Can you work these out from the model? Positions are in its coordinate system, mm. Face numbers are marked on the shaded views. A direction names the side the tool comes from. Round coordinates to 2 decimals unless told otherwise and drop trailing zeros. Loops run counter-clockwise (first coordinate to the right, second up) from the corner with the lowest first, then second, coordinate; pieces in that order, holes last. Notation, with made-up numbers: (52, 67.5) -> (60, 67.5) arc R15 ccw to (60, 79.5) -> close; hole circle Ø10 at (64, 41). An arc over 180 degrees is marked (long way). Write each question's results on one line, items separated by ' | '.
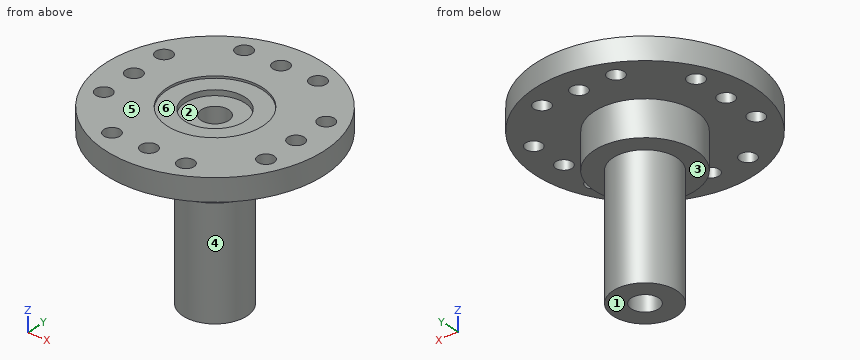
from build123d import *

# Parameters (mm, degrees)
SKETCH1_R          = 10.1727
EXTRUDE1_DEPTH     = 2.0828
SKETCH2_R          = 4.699
EXTRUDE2_DEPTH     = 3.302
SKETCH3_R          = 2.9591
EXTRUDE3_DEPTH     = 11.27
SKETCH4_R          = 4.445
CUT_EXTRUDE1_DEPTH = 0.2
SKETCH6_R          = 2.794
CUT_EXTRUDE2_DEPTH = 0.5
SKETCH7_R          = 1.27
CUT_EXTRUDE3_DEPTH = 16.9548
SKETCH8_R          = 0.762
CUT_EXTRUDE4_DEPTH = 2.0828
CIRPATTERN1_COUNT  = 4


with BuildPart() as part:
    # Sketch1 → Extrude1 (new body)
    with BuildSketch(Plane.XY):
        Circle(SKETCH1_R)
    extrude(amount=EXTRUDE1_DEPTH)

    # Sketch2 → Extrude2 (add)
    with BuildSketch(Plane(origin=(0, 0, 0), x_dir=(-1, 0, 0), z_dir=(0, 0, -1))):
        Circle(SKETCH2_R)
    extrude(amount=EXTRUDE2_DEPTH)

    # Sketch3 → Extrude3 (add)
    with BuildSketch(Plane(origin=(0, 0, -3.302), x_dir=(-1, 0, 0), z_dir=(0, 0, -1))):
        Circle(SKETCH3_R)
    extrude(amount=EXTRUDE3_DEPTH)

    # Sketch4 → Cut-Extrude1 (cut)
    with BuildSketch(Plane.XY.offset(2.0828)):
        Circle(SKETCH4_R)
    extrude(amount=-CUT_EXTRUDE1_DEPTH, mode=Mode.SUBTRACT)

    # Sketch6 → Cut-Extrude2 (cut)
    with BuildSketch(Plane.XY.offset(1.8828)):
        Circle(SKETCH6_R)
    extrude(amount=-CUT_EXTRUDE2_DEPTH, mode=Mode.SUBTRACT)

    # Sketch7 → Cut-Extrude3 (cut, through all)
    with BuildSketch(Plane.XY.offset(1.3828)):
        Circle(SKETCH7_R)
    extrude(amount=-CUT_EXTRUDE3_DEPTH, mode=Mode.SUBTRACT)

    # Sketch8 → Cut-Extrude4 (cut)
    with BuildSketch(Plane.XY.offset(2.0828)):
        with Locations((7.6327, 0)):
            Circle(SKETCH8_R)
        with Locations((7.6327, -3.4798)):
            Circle(SKETCH8_R)
        with Locations((7.6327, 3.4798)):
            Circle(SKETCH8_R)
    cut_extrude4 = extrude(amount=-CUT_EXTRUDE4_DEPTH, mode=Mode.SUBTRACT)

    # CirPattern1: Cut-Extrude4 ×4 about axis
    cirpattern1_axis = Axis((0, 0, 0), (0, 0, 1))
    for i in range(1, CIRPATTERN1_COUNT):
        add(cut_extrude4.rotate(cirpattern1_axis, i * 360 / CIRPATTERN1_COUNT), mode=Mode.SUBTRACT)


solid = part.part
1. If we section it at D-D (x = -7.25): List the corners of the cut face in (y, z) for me.
Final values:
outline: (-7.14, 0) -> (-4.14, 0) -> (-4.14, 2.08) -> (-7.14, 2.08) -> close; (-2.82, 0) -> (-0.66, 0) -> (-0.66, 2.08) -> (-2.82, 2.08) -> close; (0.66, 0) -> (2.82, 0) -> (2.82, 2.08) -> (0.66, 2.08) -> close; (4.14, 0) -> (7.14, 0) -> (7.14, 2.08) -> (4.14, 2.08) -> close
2. We'd pull the mould along X, two halves only. Please class the marked faces 4, 5 and 6: pulls with the +X half, pulls with the -X half, needs draft (parallel to the pull), parting line crosses it, or undercut.
Final values:
face 4: parting line crosses it | face 5: needs draft | face 6: undercut
3. If we section it at A-A (x = 0): State how many separate pieces and enclosed holes the cut face has, then the cut area to 3 significant figures.
Final values:
separate pieces: 4 | enclosed holes: 0 | area: 88.7 mm2
4. Will these pins go through, and if not, where does the flat tip stop? pin 1 (2 mm diameter, centred on x = -2.5, z = -5.5, fed in from +Y); pin 2 (5 mm diameter, centred on y = 3.5, z = -6, fed in from -X) (3 decimals); pin 3 (7.5 mm diameter, centred on x = 0, y = 0, fed in from +Z); pin 4 (1.2 mm diameter, centred on x = -7.63, y = 0, fed in from +Z) (3 decimals).
Final values:
pin 1: y = 2.55 | pin 2: x = -2.785 | pin 3: z = 1.88 | pin 4: through
5. If we section it at C-C (z = -12.25): List the corners of the cut face in (x, y) for me, then the cut area to 3 significant figures.
Final values:
outline: circle Ø5.92 at (0, 0); hole circle Ø2.54 at (0, 0) | area: 22.4 mm2
6. On a 3-axis mill with a long thin cutter (end or side, diameter ignored), from which of +Z, -Z, +X, -X, +Y, -Y can I reach the whole of each face in a straight line? I mean the marked faces 1, 2 and 3. Say none if no direction works.
Final values:
face 1: -Z, +X, -X, +Y, -Y | face 2: +Z | face 3: -Z
7. Please list where these lines run through material, in increasing order: line 1 (Z direction, x = -2, y = 2.5); line 2 (Z direction, x = -4.5, y = 0); line 3 (X direction, y = -0.75, z = -6). Write a range as from..to.
Final values:
line 1: -3.3..1.88 | line 2: -3.3..2.08 | line 3: -2.86..-1.02, 1.02..2.86
